Model file for the job. Use its own axes, mm. Face numbers are marked on the shaded views. A direction names the side the tool comes from. Coordinates: 2 decimals unless noted, no trailing zeros. Order: outer loops, then holes, each group sorted by start corner. A loop starts at its lowest first (then second) coordinate and runs counter-clockwise, first axis right, second up. Notation, with made-up numbers: (-13, 87.25) -> (33, 87.25) arc R26 cw to (33, 108.25) -> close; hole circle Ø5 at (52, 40). An arc over 180 degrees is marked (long way). Write item = value, one per line. Start each with the question number.
Q1. Cut at D-D, the plane y = 12.35. Give the number of separate pieces and of enclosed holes in the cut face, plus the area to 3 significant figures.
Q2. Cut at B-B, the plane z = 42. List the corners of the cut face in (x, y).
Q3. Flat gauge pins, fed straight in: pin 1 (4 mm diameter, centred on y = 18, z = 32, fed in from -X); pin 2 (8 mm diameter, centred on x = 10, y = 12.35, fed in from +Z); pin 3 (3 mm diameter, centred on x = 64.5, y = 9.5, fed in from +Z); pin 4 (0.8 mm diameter, centred on x = 3, z = 23, fed in from -Y). Where does each tip first touch, or does it go through?
Q4. 3-axis set-ups, long thin cutter, end or side, ignore diameter. For the marked faces 5, 6 and 7: which of +Z, -Z, +X, -X, +Y, -Y reach the whole face in a straight line?
Q5. Mould opens along Y. For the marked faces 1, 2, 3 and 4 say: +Y half, -Y half, draft (parallel to the pull), parting line (faces both ways), or undercut.
Q6. Cut at A-A, the plane y = 18.75. List the corners of the cut face in (x, z), plus the area to 3 significant figures.
Q7. Wall check: line 1 (X direction, y = 12.35, z = 84.25); line 2 (X direction, y = 12.35, z = 54.5); line 3 (Z direction, x = 6, y = 15). Give the ranges that are in metal, low to high. Write a range as from..to.
Q8. Cut at C-C, the plane x = 56. List the corners of the cut face in (y, z).
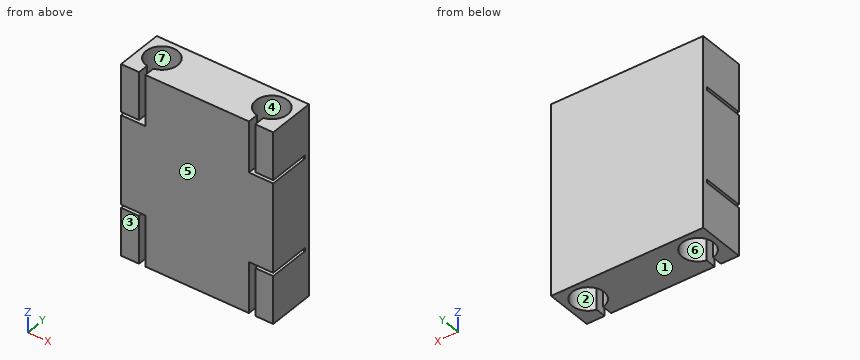
Autodesk Inventor part; units mm, degrees
ref_plane "Work Plane1" through (0, 0, 66) normal (0, 0, 1) x (1, 0, 0)
ref_plane "Work Plane2" through (0, 0, 24) normal (0, 0, -1) x (-1, 0, 0)
ref_plane "YZ Plane" through (0, 0, 0) normal (1, 0, 0) x (0, 1, 0)
sketch "Sketch1" plane through (0, 0, 0) normal (0, 0, 1) x (1, 0, 0)
  line L0 (0, 0) -> (0, 22.35)
  line L1 (0, 22.35) -> (72, 22.35)
  line L2 (72, 22.35) -> (72, 0)
  arc A0 (11.5, 5.0015) -> (8.5, 5.0015) centre (10, 12.35) ccw
  arc A1 (63.5, 5.0015) -> (60.5, 5.0015) centre (62, 12.35) ccw
  line L3 (72, 0) -> (63.5, 0)
  line L4 (63.5, 0) -> (63.5, 5.0015)
  line L5 (60.5, 5.0015) -> (60.5, 0)
  line L6 (60.5, 0) -> (11.5, 0)
  line L7 (11.5, 0) -> (11.5, 5.0015)
  line L8 (8.5, 5.0015) -> (8.5, 0)
  line L9 (8.5, 0) -> (0, 0)
  dimension "d0" = 22.35
  dimension "d1" = 72
  dimension "d2" = 15
  dimension "d4" = 10
  dimension "d5" = 10
  dimension "d6" = 10
  dimension "d7" = 3
  dimension "d8" = 3
extrude "Extrusion1" add sketch "Sketch1" along normal blind 90
ref_plane "Work Plane1" through (0, 0, 66) normal (0, 0, 1) x (1, 0, 0)
sketch "Sketch2" plane through (0, 0, 66) normal (0, 0, 1) x (1, 0, 0)
  line L0 (0, 22.35) -> (0, 0)
  line L1 (0, 0) -> (8.5, 0)
  line L2 (8.5, 0) -> (8.5, 5.0015)
  arc A0 (11.5, 5.0015) -> (8.5, 5.0015) centre (10, 12.35) ccw
  line L3 (11.5, 5.0015) -> (11.5, 0)
  line L4 (11.5, 0) -> (60.5, 0)
  line L5 (60.5, 0) -> (60.5, 5.0015)
  arc A1 (63.5, 5.0015) -> (60.5, 5.0015) centre (62, 12.35) ccw
  line L6 (63.5, 5.0015) -> (63.5, 0)
  line L7 (63.5, 0) -> (72, 0)
  line L8 (72, 0) -> (72, 22.35)
  line L9 (72, 22.35) -> (0, 22.35)
  line L10 (8.5, 0) -> (11.5, 0)
  line L11 (11.5, 0) -> (60.5, 0)
  line L12 (60.5, 0) -> (63.5, 0)
ref_plane "Work Plane2" through (0, 0, 24) normal (0, 0, -1) x (-1, 0, 0)
extrude "Extrusion2" add sketch "Sketch2" against normal up to surface (42 mm away) contours L2 A0 L3 L10 | L12 L5 A1 L6
sketch "Sketch3" plane through (0, 0, 66) normal (0, 0, 1) x (1, 0, 0)
  arc A0 (11.5, 5.0015) -> (8.5, 5.0015) centre (10, 12.35) ccw
  line L0 (60.5, 0) -> (63.5, 0)
  line L1 (63.5, 5.0015) -> (63.5, 0)
  arc A1 (63.5, 5.0015) -> (60.5, 5.0015) centre (62, 12.35) ccw
  line L2 (60.5, 0) -> (60.5, 5.0015)
  circle A2 centre (10, 12.35) radius 4.5
  circle A3 centre (62, 12.35) radius 4.5
  point P0 (0, 0)
  dimension "d15" = 9
  dimension "d16" = 9
extrude "Extrusion3" cut sketch "Sketch3" against normal up to surface (42 mm away) contours A2 | A3
sketch "Sketch4" plane through (72, 0, 0) normal (1, 0, 0) x (0, 0, -1)
  line L0 (0, 22.35) -> (0, 0)
  line L1 (0, 22.35) -> (-90, 22.35)
  line L2 (-90, 0) -> (-90, 22.35)
  line L3 (0, 0) -> (-90, 0)
  line L4 (-66, 5.0015) -> (-66, 19.85)
  line L5 (-24, 19.85) -> (-24, 5.0015)
  line L6 (-66, 19.85) -> (-67.5, 19.85)
  line L7 (-90, 19.85) -> (-66, 19.85)
  line L8 (-67.5, 19.85) -> (-67.5, 0)
  line L9 (0, 0) -> (-90, 0)
  line L10 (-66, 5.0015) -> (-66, 0)
  line L11 (-66, 0) -> (-66, 5.0015)
  line L12 (-24, 19.85) -> (-22.5, 19.85)
  line L13 (-24, 19.85) -> (0, 19.85)
  line L14 (-22.5, 19.85) -> (-22.5, 0)
  line L15 (-24, 5.0015) -> (-24, 0)
  line L16 (-24, 5.0015) -> (-24, 0)
  dimension "d19" = 1.5
  dimension "d20" = 1.5
extrude "Extrusion4" cut sketch "Sketch4" against normal blind 10 contours L14 L3 L15 L5 L12 | L6 L4 L10 L3 L8
sketch "Sketch5" plane through (0, 0, 0) normal (-1, 0, 0) x (0, 0, 1)
  line L0 (0, 0) -> (90, 0)
  line L1 (67.5, 0) -> (67.5, 19.85)
  line L2 (67.5, 19.85) -> (66, 19.85)
  line L3 (66, 19.85) -> (66, 0)
  line L4 (24, 0) -> (24, 19.85)
  line L5 (24, 19.85) -> (22.5, 19.85)
  line L6 (22.5, 19.85) -> (22.5, 0)
extrude "Extrusion5" cut sketch "Sketch5" against normal blind 10
properties part number "XCarriageHexagon"
Here are the results:
q1.separate_pieces = 7
q1.enclosed_holes = 0
q1.area = 4,270 mm²
q2.outline = (0, 0) -> (72, 0) -> (72, 22.35) -> (0, 22.35) -> close; hole circle Ø9 at (10, 12.35); hole circle Ø9 at (62, 12.35)
q3.pin_1 = 0
q3.pin_2 = through
q3.pin_3 = 66
q3.pin_4 = 19.85
q4.face_5 = +Z, -Z, +X, -X, -Y
q4.face_6 = -Z
q4.face_7 = +Z
q5.face_1 = draft
q5.face_2 = undercut
q5.face_3 = -Y half
q5.face_4 = undercut
q6.outline = (0, 0) -> (6.09, 0) -> (6.09, 22.5) -> (0, 22.5) -> close; (0, 24) -> (13.91, 24) -> (13.91, 0) -> (58.09, 0) -> (58.09, 24) -> (72, 24) -> (72, 66) -> (58.09, 66) -> (58.09, 90) -> (13.91, 90) -> (13.91, 66) -> (0, 66) -> close; (0, 67.5) -> (6.09, 67.5) -> (6.09, 90) -> (0, 90) -> close; (65.91, 0) -> (72, 0) -> (72, 22.5) -> (65.91, 22.5) -> close; (65.91, 67.5) -> (72, 67.5) -> (72, 90) -> (65.91, 90) -> close
q6.area = 5,690 mm²
q7.line_1 = 0..2.5, 17.5..54.5, 69.5..72
q7.line_2 = 0..5.5, 14.5..57.5, 66.5..72
q7.line_3 = 24..66
q8.outline = (0, 0) -> (7.85, 0) -> (7.85, 24) -> (16.85, 24) -> (16.85, 0) -> (22.35, 0) -> (22.35, 90) -> (16.85, 90) -> (16.85, 66) -> (7.85, 66) -> (7.85, 90) -> (0, 90) -> close
